```python
from build123d import *

# Parameters (mm, degrees)
SKETCH1_W           = 130
SKETCH1_H           = 130
SKETCH1_W_2         = 30
SKETCH1_H_2         = 30
BOSS_EXTRUDE1_DEPTH = 3
CUT_EXTRUDE1_DEPTH  = 3
CUT_EXTRUDE2_DEPTH  = 3


with BuildPart() as part:
    # Sketch1 → Boss-Extrude1 (new body)
    with BuildSketch(Plane(origin=(0, 0, 0), x_dir=(1, 0, 0), z_dir=(0, 1, 0))):
        Rectangle(SKETCH1_W, SKETCH1_H)
        Polygon((-55, 40.857864376), (-25, 10.857864376), (-25, -10.857864376), (-55, -40.857864376), align=None, mode=Mode.SUBTRACT)
        Polygon((-40.857864376, -55), (-10.857864376, -25), (10.857864376, -25), (40.857864376, -55), align=None, mode=Mode.SUBTRACT)
        Polygon((55, -40.857864376), (25, -10.857864376), (25, 10.857864376), (55, 40.857864376), align=None, mode=Mode.SUBTRACT)
        Polygon((40.857864376, 55), (10.857864376, 25), (-10.857864376, 25), (-40.857864376, 55), align=None, mode=Mode.SUBTRACT)
        Rectangle(SKETCH1_W_2, SKETCH1_H_2, mode=Mode.SUBTRACT)
    extrude(amount=BOSS_EXTRUDE1_DEPTH)

    # Sketch2 → Cut-Extrude1 (cut)
    with BuildSketch(Plane(origin=(0, 3, 0), x_dir=(1, 0, 0), z_dir=(0, 1, 0))):
        with BuildLine():
            ThreePointArc((-55.8, 57.5), (-58.702081528, 58.702081528), (-57.5, 55.8))
            Line((-57.5, 55.8), (-57.5, 57.5))
            Line((-57.5, 57.5), (-55.8, 57.5))
        make_face()
        with BuildLine():
            Line((-57.5, 57.5), (-57.5, 55.8))
            ThreePointArc((-57.5, 55.8), (-56.297918472, 56.297918472), (-55.8, 57.5))
            Line((-55.8, 57.5), (-57.5, 57.5))
        make_face()
        with BuildLine():
            Line((-57.5, -55.8), (-57.5, -57.5))
            Line((-57.5, -57.5), (-55.8, -57.5))
            ThreePointArc((-55.8, -57.5), (-56.297918472, -56.297918472), (-57.5, -55.8))
        make_face()
        with BuildLine():
            Line((-55.8, -57.5), (-57.5, -57.5))
            Line((-57.5, -57.5), (-57.5, -55.8))
            ThreePointArc((-57.5, -55.8), (-58.702081528, -58.702081528), (-55.8, -57.5))
        make_face()
        with BuildLine():
            ThreePointArc((57.5, -55.8), (56.297918472, -56.297918472), (55.8, -57.5))
            Line((55.8, -57.5), (57.5, -57.5))
            Line((57.5, -57.5), (57.5, -55.8))
        make_face()
        with BuildLine():
            Line((57.5, -57.5), (55.8, -57.5))
            ThreePointArc((55.8, -57.5), (57.5, -59.2), (59.2, -57.5))
            ThreePointArc((59.2, -57.5), (58.702081528, -56.297918472), (57.5, -55.8))
            Line((57.5, -55.8), (57.5, -57.5))
        make_face()
        with BuildLine():
            ThreePointArc((55.8, 57.5), (56.297918472, 56.297918472), (57.5, 55.8))
            Line((57.5, 55.8), (57.5, 57.5))
            Line((57.5, 57.5), (55.8, 57.5))
        make_face()
        with BuildLine():
            Line((57.5, 57.5), (57.5, 55.8))
            ThreePointArc((57.5, 55.8), (58.702081528, 56.297918472), (59.2, 57.5))
            ThreePointArc((59.2, 57.5), (57.5, 59.2), (55.8, 57.5))
            Line((55.8, 57.5), (57.5, 57.5))
        make_face()
    extrude(amount=-CUT_EXTRUDE1_DEPTH, mode=Mode.SUBTRACT)

    # Sketch3 → Cut-Extrude2 (cut)
    with BuildSketch(Plane(origin=(0, 3, 0), x_dir=(1, 0, 0), z_dir=(0, 1, 0))):
        with BuildLine():
            Line((-22.5, -20.8), (-22.5, -22.5))
            Line((-22.5, -22.5), (-20.8, -22.5))
            ThreePointArc((-20.8, -22.5), (-21.297918472, -21.297918472), (-22.5, -20.8))
        make_face()
        with BuildLine():
            Line((-20.8, -22.5), (-22.5, -22.5))
            Line((-22.5, -22.5), (-22.5, -20.8))
            ThreePointArc((-22.5, -20.8), (-23.702081528, -23.702081528), (-20.8, -22.5))
        make_face()
        with BuildLine():
            ThreePointArc((-20.8, 22.5), (-23.702081528, 23.702081528), (-22.5, 20.8))
            Line((-22.5, 20.8), (-22.5, 22.5))
            Line((-22.5, 22.5), (-20.8, 22.5))
        make_face()
        with BuildLine():
            Line((-22.5, 22.5), (-22.5, 20.8))
            ThreePointArc((-22.5, 20.8), (-21.297918472, 21.297918472), (-20.8, 22.5))
            Line((-20.8, 22.5), (-22.5, 22.5))
        make_face()
        with BuildLine():
            ThreePointArc((22.5, -20.8), (21.297918472, -21.297918472), (20.8, -22.5))
            Line((20.8, -22.5), (22.5, -22.5))
            Line((22.5, -22.5), (22.5, -20.8))
        make_face()
        with BuildLine():
            Line((22.5, -22.5), (20.8, -22.5))
            ThreePointArc((20.8, -22.5), (22.5, -24.2), (24.2, -22.5))
            ThreePointArc((24.2, -22.5), (23.702081528, -21.297918472), (22.5, -20.8))
            Line((22.5, -20.8), (22.5, -22.5))
        make_face()
        with BuildLine():
            ThreePointArc((20.8, 22.5), (21.297918472, 21.297918472), (22.5, 20.8))
            Line((22.5, 20.8), (22.5, 22.5))
            Line((22.5, 22.5), (20.8, 22.5))
        make_face()
        with BuildLine():
            Line((22.5, 22.5), (22.5, 20.8))
            ThreePointArc((22.5, 20.8), (23.702081528, 21.297918472), (24.2, 22.5))
            ThreePointArc((24.2, 22.5), (22.5, 24.2), (20.8, 22.5))
            Line((20.8, 22.5), (22.5, 22.5))
        make_face()
    extrude(amount=-CUT_EXTRUDE2_DEPTH, mode=Mode.SUBTRACT)


solid = part.part
```
Build history of the part. All positions in model axes, mm. A direction names the side the tool comes from. Give positions to 0.01 mm unless a question says otherwise; leave off trailing zeros. Order: outer loops, then holes, each group sorted by start corner. A loop starts at its lowest first (then second) coordinate and runs counter-clockwise, first axis right, second up. Notation, with made-up numbers: M -34.75,76 L 4.25,76 A19 cw 4.25,87 Z; hole C 16.5,-3 d10. An arc over 180 degrees is marked long. Write item = value, one per line. Start each with the question number.
(1) Which spindle directions (+Z, -Z, +X, -X, +Y, -Y) get a long thin tool onto all of the face, cutting with end or side? Do faces 1 (the flat face through (-25.65, 1.48, -39.79)), 2 (the flat face through (-0.9, 3, -15.4)). Say none if no direction does.
(2) Probe L1, parallel to Z at x = 3.5, y = 2.65; L2, parallel to Z at x = -57.5, y = 1.25. List the from-to ranges inside material, lowest first. Write a range as [from, to].
(3) Slice it at D-D on z = -44.5. Write the cut outline in (x, y).
(4) Slice it at A-A on z = 29.5. Write the cut outline in (x, y).
(5) Slice it at B-B on z = 51.5. Write the cut outline in (x, y).
(6) Slice it at C-C on y = 0.6. State how many separate pieces and enclosed holes the cut face has, plus the area to 3 significant figures.
(7) Two-plate mould, pull along X, no slides. Class faces 3 (the flat face through (-26.07, 1.48, 40.21)), 4 (the flat face through (65, 1, 1)), 5 (the flat face through (-1, 1, -65)): released by +X, released by -X, zero draft, split by the parting line, or undercut.
Responses:
q1.face_1 = +Y, -Y
q1.face_2 = +Z, -Z, +X, -X, +Y
q2.L1 = [-65, -55], [-25, -15], [15, 25], [55, 65]
q2.L2 = [-65, -59.2], [-55.8, 55.8], [59.2, 65]
q3.outline = M -65,0 L -30.36,0 L -30.36,3 L -65,3 Z; M 30.36,0 L 65,0 L 65,3 L 30.36,3 Z
q4.outline = M -65,0 L -55,0 L -55,3 L -65,3 Z; M -43.64,0 L -15.36,0 L -15.36,3 L -43.64,3 Z; M 15.36,0 L 43.64,0 L 43.64,3 L 15.36,3 Z; M 55,0 L 65,0 L 65,3 L 55,3 Z
q5.outline = M -65,0 L -37.36,0 L -37.36,3 L -65,3 Z; M 37.36,0 L 65,0 L 65,3 L 37.36,3 Z
q6.separate_pieces = 1
q6.enclosed_holes = 13
q6.area = 9,720 mm2
q7.face_3 = undercut
q7.face_4 = released by +X
q7.face_5 = zero draft
